Build history of the part. All positions in model axes, mm. A direction names the side the tool comes from. Round coordinates to 2 decimals unless told otherwise and drop trailing zeros. Write each loop counter-clockwise with the first axis right and the second up, starting at its lowest first coordinate (ties: lowest second). Pieces come first, ordered by that corner, then holes. Notation, with made-up numbers: (35.5, -33.75) - (53.5, -33.75) arc R22 cw to (53.5, 4.25) - close; hole circle Ø7 at (36, -10.5). An arc over 180 degrees is marked (long way). One line per question, with ' | ' between items.
from build123d import *

# Parameters (mm, degrees)
F0_W     = 200
F0_H     = 450
F1_DEPTH = 2


with BuildPart() as f1:
    # F0 (on Top) → F1 (new body)
    with BuildSketch(Plane.XY):
        Polygon((-47.865819, 70), (-47.865819, 0), (152.134181, 0), (152.134181, 70), (122.134181, 70), (102.134181, 50), (82.134181, 70), (22.134181, 70), (2.134181, 50), (-17.865819, 70), align=None)
        with Locations((52.134181, -225)):
            Rectangle(F0_W, F0_H)
        Polygon((152.134181, -450), (-47.865819, -450), (-47.865819, -520), (-17.865819, -520), (2.134181, -500), (22.134181, -520), (82.134181, -520), (102.134181, -500), (122.134181, -520), (152.134181, -520), align=None)
    extrude(amount=F1_DEPTH)


solid = f1.part
Q1. Drill centre lines: L1, parallel to Y at x = 87, z = 1.25; L2, parallel to Y at x = 83, z = 1.25. Where is each one in solid material? Low to high. Write a range as from..to.
Found:
L1: -515.13..65.13 | L2: -519.13..69.13
Q2. Pull direction X, two halves, no side cores. Call faces 4 (the flat face through (-8.006, -510.14, 0.986)), 5 (the flat face through (111.994, -509.86, 0.986)), 6 (the flat face through (51, -221, 0)): +X half, -X half, draft (parallel to the pull), parting line (faces both ways), or undercut.
Found:
face 4: undercut | face 5: undercut | face 6: draft
Q3. Which spindle directions (+Z, -Z, +X, -X, +Y, -Y) get a long thin tool onto all of the face, cutting with end or side? Do faces 1 (the flat face through (51, -221, 2)), 2 (the flat face through (-7.726, 59.86, 0.986)), 3 (the flat face through (91.994, -510.14, 0.986)). Say none if no direction does.
Found:
face 1: +Z, +X, -X, +Y, -Y | face 2: +Z, -Z, +Y | face 3: +Z, -Z, -Y
Q4. Saw through at A-A, the plane x = 88.5. List the corners of the cut face in (y, z), then the cut area to 3 significant figures.
Found:
outline: (-513.63, 0) - (63.63, 0) - (63.63, 2) - (-513.63, 2) - close | area: 1,150 mm^2
